Autodesk Inventor part; units mm, degrees
ref_plane "Work Plane1" through (0, 6.35, 0) normal (0, 1, 0) x (-1, 0, 0)
ref_plane "YZ Plane" through (0, 0, 0) normal (1, 0, 0) x (0, 1, 0)
ref_plane "XZ Plane" through (0, 0, 0) normal (0, 1, 0) x (-1, 0, 0)
sketch "Sketch1" plane through (0, 0, 0) normal (0, 0, 1) x (1, 0, 0)
  circle A0 centre (0, 0) radius 6.35
  dimension "d0" = 12.7
extrude "Extrusion1" add sketch "Sketch1" along normal blind 95.25
sketch "Sketch2" plane through (0, 0, 95.25) normal (0, 0, 1) x (1, 0, 0)
  circle A0 centre (0, 0) radius 6.35
hole "Hole1" at (0, 0, 95.25) direction (0, 0, -1) diameter 6.9088 depth 19.05 tip angle 118
ref_plane "Work Plane1" through (0, 6.35, 0) normal (0, 1, 0) x (-1, 0, 0)
sketch "Sketch3" plane through (0, 6.35, 0) normal (0, 1, 0) x (-1, 0, 0)
  line L0 (-6.35, 0) -> (6.35, 0)
  line L1 (-6.35, 95.25) -> (6.35, 95.25)
  line L2 (-6.35, 0) -> (6.35, 0)
  point P0 (0, 20.25)
  dimension "d18" = 75
hole "Hole2" at (0, 6.35, 20.25) direction (0, -1, 0) diameter 4.917 end through all
sketch "Sketch4" plane through (0, 0, 0) normal (0, 0, -1) x (-1, 0, 0)
  circle A0 centre (0, 0) radius 6.35
hole "Hole3" at (0, 0, 0) direction (0, 0, 1) diameter 3.9624 depth 6.35 tip angle 118
properties part number "PWTR-0037" material "Stainless Steel, 303"
The listing builds one solid part. Answer for the finished solid, in the listing's coordinates (mm). A direction names the side the tool comes from. Coordinates: 2 decimals unless noted, no trailing zeros. Write each loop counter-clockwise with the first axis right and the second up, starting at its lowest first coordinate (ties: lowest second). Pieces come first, ordered by that corner, then holes. Notation, with made-up numbers: (-20, 27.25) -> (15, 27.25) arc R20 ccw to (15, 41.25) -> close; hole circle Ø5 at (78.25, -1.5). An arc over 180 degrees is marked (long way). Write each question's results on one line, items separated by ' | '. Start each with the question number.
1) For a pull along X with two mould halves and no side action, classify faces 3 (the conical face through (-0.34, -0.07, 7.33)), 4 (the cylindrical face through (-3.425, 0.45, 85.592)), 5 (the flat face through (3, -3, 95.25)), 6 (the cylindrical face through (-1.38, 6.2, 46.96)) as +X half, -X half, draft (parallel to the pull), parting line (faces both ways), or undercut.
2) Flat-ended cylindrical pins translate along their axes: pin 1 Ø4.5 at (x, y) = (0, 0) entering from +Z; pin 2 Ø5 at (x, z) = (-5, 58) entering from +Y; pin 3 Ø4 at (y, z) = (-5, 16) entering from +X. Find the tip coordinate at first contact, or state that the pin passes through.
3) Straight lines are drawn through the part: probe 1 along Y at (x, z) = (0, 78); probe 2 along Z at (x, y) = (-2.25, 1.5); probe 3 along Z at (x, y) = (0, 0.25). For each, find the intervals that lie inside material, in ascending order.
4) A cutting plane is placed at B-B (z = 20.25). Determine the outline of the cut face in (x, y).
5) A tool of negligible diameter and unlimited length cuts with its end or side. For faces 1 (the cylindrical face through (-0.108, -0.089, 17.794)), 2 (the cylindrical face through (-1.964, -0.258, 3.219)), from which of +Z, -Z, +X, -X, +Y, -Y can it reach the whole face along a straight path? Write none if from no direction.
6) A cutting plane is placed at A-A (y = 5.5). Determine the outline of the cut face in (x, z), then the cut area to 3 significant figures.
7) A cutting plane is placed at C-C (z = 65.5). Determine the outline of the cut face in (x, y), then the cut area to 3 significant figures.
8) A cutting plane is placed at D-D (x = 4.75). Determine the outline of the cut face in (y, z), then the cut area to 3 significant figures.
Values follow:
1) face 3: undercut | face 4: undercut | face 5: draft | face 6: parting line
2) pin 1: z = 75.48 | pin 2: y = 5.84 | pin 3: x = 5.6
3) probe 1: -6.35 to -3.45, 3.45 to 6.35 | probe 2: 0 to 19.26, 21.24 to 75.75 | probe 3: 7.39 to 17.79, 22.71 to 74.27
4) outline: (-2.46, -5.85) -> (-2.46, 5.85) arc R6.35 ccw to start; (2.46, -5.85) arc R6.35 ccw to (2.46, 5.85) -> close
5) face 1: +Y, -Y | face 2: -Z
6) outline: (-3.17, 0) -> (3.17, 0) -> (3.17, 95.25) -> (-3.17, 95.25) -> close; hole circle Ø4.92 at (0, 20.25) | area: 586 mm²
7) outline: circle Ø12.7 at (0, 0) | area: 127 mm²
8) outline: (-4.21, 0) -> (4.21, 0) -> (4.21, 95.25) -> (-4.21, 95.25) -> close | area: 803 mm²
